Autodesk Inventor part; units mm, degrees
ref_plane "Work Plane1" through (0, 0, 0) normal (0, 0, 1) x (1, 0, 0)
ref_plane "Work Plane2" through (0, 0, 76.4) normal (0, 0, -1) x (-1, 0, 0)
ref_plane "Work Plane4" through (0, 0, 38.2) normal (0, 0, -1) x (-1, 0, 0)
ref_plane "Work Plane1" through (0, 0, 0) normal (0, 0, 1) x (1, 0, 0)
sketch "Sketch1" plane through (0, 0, 0) normal (0, 0, 1) x (1, 0, 0)
  spline S0 degree 3 poles (-17.5035, -43.75) (9.5564, -35.6427) (30.0035, -17.8707) (22.4965, 16.6912) knots 1 1 1 1 2 2 2 2
  line L0 (22.4965, 16.6912) -> (-1.9986, 25.6067)
  line L1 (-17.5035, 14.75) -> (-17.5035, -43.75)
  line L2 (-3.0246, 22.7876) -> (19.8959, 14.4452)
  line L3 (-14.5035, -39.6343) -> (-14.5035, 14.75)
  line L4 (19.8959, 14.4452) -> (19.8959, 17.6377)
  line L5 (-14.5035, -39.6343) -> (-17.5035, -40.6309)
  spline S1 degree 5 poles (19.896, 14.4452) (20.6656, 10.4799) (21.1568, 6.4613) (21.3154, 2.402) (20.7956, -5.2165) (18.5576, -12.5026) (17.0978, -15.7703) (13.3907, -21.8782) (8.4101, -27.002) (5.6606, -29.2971) (0.173, -33.1415) (-5.7852, -36.2005) (-8.6407, -37.4765) (-11.551, -38.6165) (-14.5035, -39.6343) knots 0 0 0 0 0 0 0.283225 0.283225 0.283225 0.531381 0.531381 0.531381 0.781029 0.781029 0.781029 1 1 1 1 1 1
  point P0 (0, 0)
  dimension "d0" = 3
  dimension "d1" = 3.1612
extrude "Extrusion1" add sketch "Sketch1" along normal blind 76.4
ref_plane "Work Plane2" through (0, 0, 76.4) normal (0, 0, -1) x (-1, 0, 0)
sketch "Sketch2" plane through (0, 0, 76.4) normal (0, 0, -1) x (-1, 0, 0)
  circle A0 centre (12.5035, -33.75) radius 1.25
  line L0 (14.5035, -39.6343) -> (17.5035, -40.6309)
  line L1 (17.5035, -40.6309) -> (14.5806, -32.0992)
  line L2 (6.1137, -36.5355) -> (12.1128, -30.6255)
  circle A1 centre (12.5035, -33.75) radius 2.5
  spline S0 degree 5 poles (-19.8959, 14.4452) (-20.6656, 10.4799) (-21.1568, 6.4613) (-21.3154, 2.402) (-20.7956, -5.2165) (-18.5576, -12.5026) (-17.0978, -15.7703) (-13.3907, -21.8782) (-8.4101, -27.002) (-5.6606, -29.2971) (-0.173, -33.1415) (5.7852, -36.2005) (8.6407, -37.4765) (11.551, -38.6165) (14.5035, -39.6343) knots 0 0 0 0 0 0 0.283225 0.283225 0.283225 0.531381 0.531381 0.531381 0.781029 0.781029 0.781029 1 1 1 1 1 1
  point P0 (0, 0)
  point P1 (14.8685, -32.9397)
  point P2 (10.749, -31.9691)
  point P3 (6.3139, -36.3383)
  dimension "d4" = 5
extrude "Extrusion2" add sketch "Sketch2" along normal blind 2
ref_plane "Work Plane3" through (0, 0, 76.4) normal (0, 0, -1) x (-1, 0, 0)
sketch "Sketch3" plane through (0, 0, 76.4) normal (0, 0, -1) x (-1, 0, 0)
  circle A0 centre (-16.1637, 12.079) radius 1.25
  circle A1 centre (-16.1637, 12.079) radius 2.5
  line L0 (-19.8959, 17.6377) -> (-19.8959, 14.4452)
  line L1 (-14.7586, 14.1468) -> (-19.8959, 17.6377)
  line L2 (-16.1637, 9.579) -> (-20.6272, 9.8544)
  spline S0 degree 5 poles (-19.8959, 14.4452) (-20.6656, 10.4799) (-21.1568, 6.4613) (-21.3154, 2.402) (-20.7956, -5.2165) (-18.5576, -12.5026) (-17.0978, -15.7703) (-13.3907, -21.8782) (-8.4101, -27.002) (-5.6606, -29.2971) (-1.6234, -32.1254) (2.6686, -34.5287) (3.8695, -35.1608) (5.0852, -35.7635) (6.3139, -36.3383) knots 0 0 0 0 0 0 0.323263 0.323263 0.323263 0.6065 0.6065 0.6065 0.891438 0.891438 0.891438 1 1 1 1 1 1
  point P0 (0, 0)
  dimension "d7" = 5
extrude "Extrusion3" add sketch "Sketch3" along normal blind 2
ref_plane "Work Plane4" through (0, 0, 38.2) normal (0, 0, -1) x (-1, 0, 0)
mirror "Mirror1" about plane through (0, 0, 38.2) normal (0, 0, -1) of "Extrusion3", "Extrusion2"
properties part number "clamsheel sheet surface" material "ABS Plastic"
Build history of the part. All positions in model axes, mm. A direction names the side the tool comes from. Round coordinates to 2 decimals unless told otherwise and drop trailing zeros. Write each question's results on one line, items separated by ' | '. Start each with the question number.
Item 1: Drop flat-ended pins along their axis: P1, Ø1.5, axis at x = -12.5, y = -33.75, coming from the -Z side; P2, Ø3.5, axis at x = 16, y = 13.5, coming from the -Z side; P3, Ø5, axis at y = -16, z = 26, coming from the -X side; P4, Ø5, axis at y = -3, z = 19.5, coming from the +X side. Give the stop position or say it passes through.
Item 2: Which spindle directions (+Z, -Z, +X, -X, +Y, -Y) get a long thin tool onto all of the face, cutting with end or side? Do faces 5 (the face through (-12, -36, 74.4)), 6 (the face through (-8.563, -34.123, 0.986)), 7 (the face through (18.364, 9.715, 75.414)). Say none if no direction does.
Item 3: Mould opens along Y. For faces 1 (the face through (-13.08, -34.86, 0.99)), 2 (the face through (17.363, 15.917, 0.986)), 3 (the face through (19.896, 16, 38)), 4 (the face through (18.43, 9.72, 0.99)) say: pulls with the +Y half, pulls with the -Y half, needs draft (parallel to the pull), parting line crosses it, or undercut.
Item 4: Wall check: L1, parallel to X at y = -33, z = 75; L2, parallel to Z at x = -14.5, y = -39; L3, parallel to Y at x = 1.5, z = 59. Give the ranges that are in metal, low to high. Write a range as [from, to].
Results are:
1) P1: passes through | P2: stops at z = 0 | P3: stops at x = 15.26 | P4: stops at x = 23.95
2) face 5: -X, +Y | face 6: +Z, -Z, +Y | face 7: +Z, -Z
3) face 1: undercut | face 2: pulls with the +Y half | face 3: needs draft | face 4: undercut
4) L1: x = [-14.89, -13.5], [-11.5, -9.7], [-0.04, 5.42] | L2: z = [0, 2], [74.4, 76.4] | L3: y = [-35.58, -32.04]
